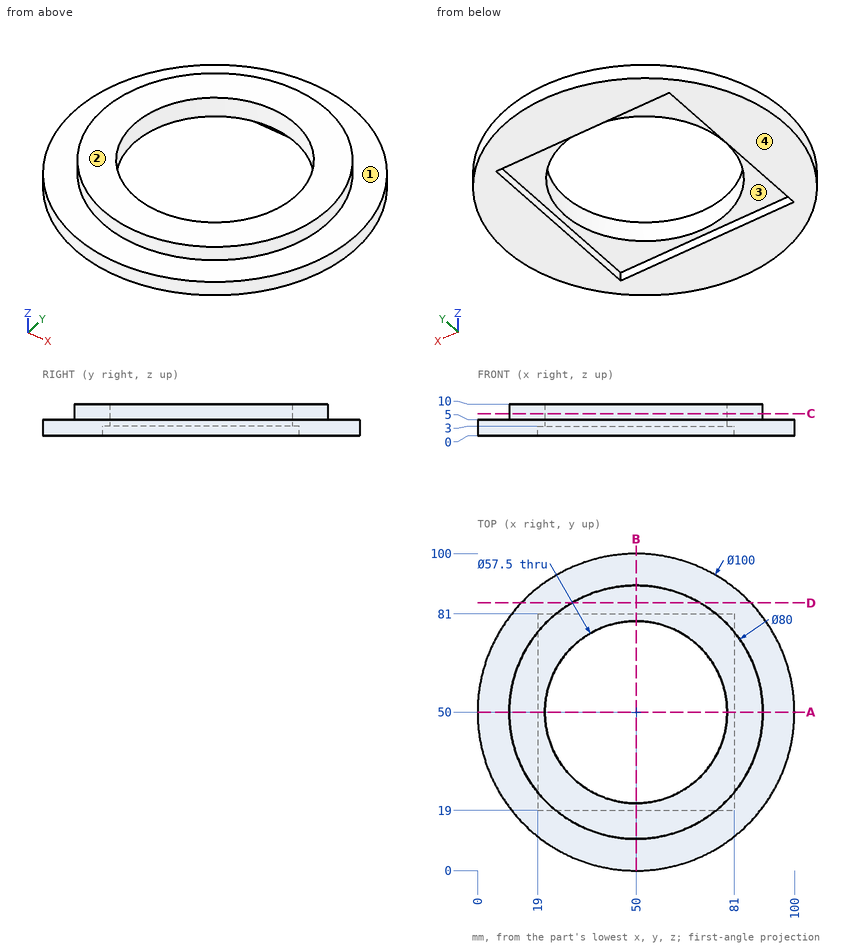
Answer from the drawing. Dimensions are ordinates in mm from the lowest x, y and z of the part. A direction names the side the tool comes from. Give positions to 0.01 mm unless a question says otherwise; leave off trailing zeros. Order: outer loops, then holes, each group sorted by start corner. A loop starts at its lowest first (then second) coordinate and runs counter-clockwise, first axis right, second up.
(1) Straight lines are drawn through the part: L1, parallel to Y at x = 50, z = 8.75; L2, parallel to Z at x = 43, y = 91. For each, find the intervals that lie inside material, in ascending order.
(2) Find section D-D (y = 84.5). Give the vertices of the cut face in (x, z).
(3) Find section C-C (z = 7). Give the vertices of the cut face in (x, y), plus the area to 3 significant figures.
(4) For a pull along X with two mould halves and no side action, classify the marked faces 3 and 4 as released by +X, released by -X, zero draft, split by the parting line, or undercut.
(5) For the marked faces 1 and 2, determine the directions among +Z, -Z, +X, -X, +Y, -Y from which every point of the face is accessible in a straight line to the end or side of a thin tool.
(6) Find section A-A (y = 50). Give the vertices of the cut face in (x, z).
(7) Given pin 1 (3.5 mm diameter, centred on x = 34.5, z = 2, fed in from -Y); pin 2 (2.5 mm diameter, centred on y = 54.5, z = 2, fed in from -X); pin 3 (4 mm diameter, centred on x = 87.5, z = 3, fed in from -Y), each flat-ended and moving along its own axis, determine where each tip first touches the part or whether it passes through.
Result sheet:
1. L1: y = 10 to 21.25, 78.75 to 90
1. L2: z = 0 to 5
2. outline: (13.81, 0) - (86.19, 0) - (86.19, 5) - (70.24, 5) - (70.24, 10) - (29.76, 10) - (29.76, 5) - (13.81, 5) - close
3. outline: circle Ø80 at (50, 50); hole circle Ø57.5 at (50, 50)
3. area: 2,430 mm2
4. face 3: undercut
4. face 4: zero draft
5. face 1: +Z
5. face 2: +Z, +X, -X, +Y, -Y
6. outline: (0, 0) - (19, 0) - (19, 3) - (21.25, 3) - (21.25, 10) - (10, 10) - (10, 5) - (0, 5) - close; (78.75, 3) - (81, 3) - (81, 0) - (100, 0) - (100, 5) - (90, 5) - (90, 10) - (78.75, 10) - close
7. pin 1: stops at y = 1.93
7. pin 2: stops at x = 0.11
7. pin 3: stops at y = 14.79
